Here's how the part is built. I have some questions about the finished solid (model axes, mm). Round coordinates to 2 decimals unless told otherwise and drop trailing zeros. Write each loop counter-clockwise with the first axis right and the second up, starting at its lowest first coordinate (ties: lowest second). Pieces come first, ordered by that corner, then holes. Notation, with made-up numbers: (-36.75, 8) - (14.25, 8) arc R20 ccw to (14.25, 34) - close; hole circle Ø7 at (8.25, 62.25). An arc over 180 degrees is marked (long way). Write item = value, one per line. Start each with the question number.
Item 1: If we section it at C-C (z = 1.45): Give the number of separate pieces and of enclosed holes in the cut face, and give its area (3 significant figures).
Item 2: If we section it at B-B (y = -61.5): Please give me the cut outline in (x, z).
Item 3: For P1, Ø2.5, axis at x = 1.46, y = 102.81, coming from the +Z side, with a flat end and sliding along its axis, tell me the tip position at first contact or that it passes through.
Item 4: If I drill on line 1 along X through (y, z) = (56.5, 0.6); line 2 along X through (y, z) = (-90.5, 0.7); line 3 along Y through (x, z) = (-73, 0.85), over which ranges is the centre line in solid material (lowest first)? Write a range as [from, to].
Item 5: If we section it at A-A (x = 50.5): Please give me the cut outline in (y, z), and give its area (3 significant figures).
```python
from build123d import *

# Parameters (mm, degrees)
SKETCH_1_W          = 4
SKETCH_1_H          = 1.5
EXTRUDE_1_DEPTH     = 2
SKETCH_3_R          = 1.5
SKETCH_3_R_2        = 1.65
SKETCH_3_W          = 8.03
SKETCH_3_H          = 4.03
SKETCH_3_W_2        = 4.03
SKETCH_3_H_2        = 8.03
CUT_EXTRUDE_2_DEPTH = 4
SKETCH_7_R          = 3
CUT_EXTRUDE_3_DEPTH = 10
SKETCH_8_W          = 220
SKETCH_8_H          = 220
CUT_EXTRUDE_4_DEPTH = 4


with BuildPart() as part:
    # 草图1 → 凸台-拉伸1 (new body)
    with BuildSketch(Plane.XY):
        Polygon((151.457142857, -41.187142857), (151.457142857, 108.812857143), (-148.542857143, 108.812857143), (-148.542857143, -191.187142857), (151.457142857, -191.187142857), align=None)
        with Locations((65.457142857, 98.062857143)):
            Rectangle(SKETCH_1_W, SKETCH_1_H, mode=Mode.SUBTRACT)
        with Locations((-62.542857143, 98.062857143)):
            Rectangle(SKETCH_1_W, SKETCH_1_H, mode=Mode.SUBTRACT)
    extrude(amount=EXTRUDE_1_DEPTH)

    # 草图3 → 切除-拉伸2 (cut)
    with BuildSketch(Plane.XY.offset(2)):
        with Locations((1.457142857, -185.187142857)):
            Circle(SKETCH_3_R)
        with Locations((67.457142857, -185.187142857)):
            Circle(SKETCH_3_R)
        with Locations((-64.542857143, -185.187142857)):
            Circle(SKETCH_3_R)
        with Locations((-142.542857143, 24.812857143)):
            Circle(SKETCH_3_R)
        with Locations((-142.542857143, -41.187142857)):
            Circle(SKETCH_3_R)
        with Locations((-142.542857143, -107.187142857)):
            Circle(SKETCH_3_R)
        with Locations((67.457142857, 102.812857143)):
            Circle(SKETCH_3_R)
        with Locations((1.457142857, 102.812857143)):
            Circle(SKETCH_3_R)
        with Locations((-64.542857143, 102.812857143)):
            Circle(SKETCH_3_R)
        with Locations((145.457142857, -107.187142857)):
            Circle(SKETCH_3_R)
        with Locations((145.457142857, -41.187142857)):
            Circle(SKETCH_3_R)
        with Locations((145.457142857, 24.812857143)):
            Circle(SKETCH_3_R)
        with Locations((1.457142857, -108.687142857)):
            Circle(SKETCH_3_R_2)
        with Locations((-46.272564873, -88.916850587)):
            Circle(SKETCH_3_R_2)
        with Locations((-66.042857143, -41.187142857)):
            Circle(SKETCH_3_R_2)
        with Locations((-46.272564873, 6.542564873)):
            Circle(SKETCH_3_R_2)
        with Locations((1.457142857, 26.312857143)):
            Circle(SKETCH_3_R_2)
        with Locations((49.186850587, 6.542564873)):
            Circle(SKETCH_3_R_2)
        with Locations((68.957142857, -41.187142857)):
            Circle(SKETCH_3_R_2)
        with Locations((49.186850587, -88.916850587)):
            Circle(SKETCH_3_R_2)
        with Locations((1.457142857, -125.187142857)):
            Circle(SKETCH_3_R)
        with Locations((100.457142857, -185.187142857)):
            Rectangle(SKETCH_3_W, SKETCH_3_H)
        with Locations((34.457142857, -185.187142857)):
            Rectangle(SKETCH_3_W, SKETCH_3_H)
        with Locations((-31.542857143, -185.187142857)):
            Rectangle(SKETCH_3_W, SKETCH_3_H)
        with Locations((-97.542857143, -185.187142857)):
            Rectangle(SKETCH_3_W, SKETCH_3_H)
        with Locations((-142.542857143, 57.812857143)):
            Rectangle(SKETCH_3_W_2, SKETCH_3_H_2)
        with Locations((-142.542857143, -8.187142857)):
            Rectangle(SKETCH_3_W_2, SKETCH_3_H_2)
        with Locations((-142.542857143, -74.187142857)):
            Rectangle(SKETCH_3_W_2, SKETCH_3_H_2)
        with Locations((-142.542857143, -140.187142857)):
            Rectangle(SKETCH_3_W_2, SKETCH_3_H_2)
        with Locations((100.457142857, 102.812857143)):
            Rectangle(SKETCH_3_W, SKETCH_3_H)
        with Locations((34.457142857, 102.812857143)):
            Rectangle(SKETCH_3_W, SKETCH_3_H)
        with Locations((-31.542857143, 102.812857143)):
            Rectangle(SKETCH_3_W, SKETCH_3_H)
        with Locations((-97.542857143, 102.812857143)):
            Rectangle(SKETCH_3_W, SKETCH_3_H)
        with Locations((145.457142857, -140.187142857)):
            Rectangle(SKETCH_3_W_2, SKETCH_3_H_2)
        with Locations((145.457142857, -74.187142857)):
            Rectangle(SKETCH_3_W_2, SKETCH_3_H_2)
        with Locations((145.457142857, -8.187142857)):
            Rectangle(SKETCH_3_W_2, SKETCH_3_H_2)
        with Locations((145.457142857, 57.812857143)):
            Rectangle(SKETCH_3_W_2, SKETCH_3_H_2)
    extrude(amount=-CUT_EXTRUDE_2_DEPTH, mode=Mode.SUBTRACT)

    # 草图7 → 切除-拉伸3 (cut)
    with BuildSketch(Plane.XY.offset(2)):
        with Locations((-88.542857143, -171.187142857)):
            Circle(SKETCH_7_R)
        with Locations((91.457142857, -171.187142857)):
            Circle(SKETCH_7_R)
        with Locations((-128.542857143, 48.812857143)):
            Circle(SKETCH_7_R)
        with Locations((-128.542857143, -131.187142857)):
            Circle(SKETCH_7_R)
        with Locations((91.457142857, 88.812857143)):
            Circle(SKETCH_7_R)
        with Locations((-88.542857143, 88.812857143)):
            Circle(SKETCH_7_R)
        with Locations((131.457142857, -131.187142857)):
            Circle(SKETCH_7_R)
        with Locations((131.457142857, 48.812857143)):
            Circle(SKETCH_7_R)
    extrude(amount=-CUT_EXTRUDE_3_DEPTH, mode=Mode.SUBTRACT)

    # 草图8 → 切除-拉伸4 (cut)
    with BuildSketch(Plane.XY.offset(2)):
        with Locations((1.457142857, -41.187142857)):
            Rectangle(SKETCH_8_W, SKETCH_8_H)
    extrude(amount=-CUT_EXTRUDE_4_DEPTH, mode=Mode.SUBTRACT)


solid = part.part
```
Reply:
q1.separate_pieces = 1
q1.enclosed_holes = 39
q1.area = 40,800 mm2
q2.outline = (-148.54, 0) - (-108.54, 0) - (-108.54, 2) - (-148.54, 2) - close; (111.46, 0) - (151.46, 0) - (151.46, 2) - (111.46, 2) - close
q3.P1 = through
q4.line_1 = [-148.54, -144.56], [-140.53, -108.54], [111.46, 143.44], [147.47, 151.46]
q4.line_2 = [-148.54, -108.54], [111.46, 151.46]
q4.line_3 = [-191.19, -151.19], [68.81, 108.81]
q5.outline = (-191.19, 0) - (-151.19, 0) - (-151.19, 2) - (-191.19, 2) - close; (68.81, 0) - (108.81, 0) - (108.81, 2) - (68.81, 2) - close
q5.area = 160 mm2
